Model file for the job. Use its own axes, mm. Face numbers are marked on the shaded views. Coordinates: 2 decimals unless noted, no trailing zeros. Order: outer loops, then holes, each group sorted by start corner. A loop starts at its lowest first (then second) coordinate and runs counter-clockwise, first axis right, second up.
from build123d import *

# Parameters (mm, degrees)
CROQUIS1_W                         = 431.038
CROQUIS1_H                         = 381
BRIDA_BASE1_DEPTH                  = 1.524
CORTAR_EXTRUIR1_REACH              = 289.647
CROQUIS6_W                         = 4.826
CROQUIS6_H                         = 4.826
BRIDA_DE_ARISTA1_STRIP_W           = 9.144
BRIDA_DE_ARISTA1_STRIP_H           = 1.524
BRIDA_DE_ARISTA1_STRIP_CUT_DEPTH   = 426.212
BRIDA_DE_ARISTA1_STRIP_2_W         = 9.144
BRIDA_DE_ARISTA1_STRIP_2_H         = 1.524
BRIDA_DE_ARISTA1_STRIP_CUT_2_DEPTH = 426.212
BRIDA_DE_ARISTA1_STRIP_3_W         = 9.144
BRIDA_DE_ARISTA1_STRIP_3_H         = 1.524
BRIDA_DE_ARISTA1_STRIP_CUT_3_DEPTH = 371.348
BRIDA_DE_ARISTA1_DEPTH             = 426.212
BRIDA_DE_ARISTA1_BEND_DEPTH        = 426.212
BRIDA_DE_ARISTA1_BEND_2_DEPTH      = 371.348
CORTAR_EXTRUIR2_REACH              = 290.088
CROQUIS16_R                        = 3.9624
CROQUIS16_R_2                      = 2.8956
CROQUIS16_R_3                      = 2.413


# Sheet-metal steps are written as plain solids
with BuildPart() as part:
    # Croquis1 → Brida base1 (new body)
    with BuildSketch(Plane.XY):
        Rectangle(CROQUIS1_W, CROQUIS1_H)
    extrude(amount=-BRIDA_BASE1_DEPTH)

    # Croquis6 → Cortar-Extruir1 (cut, up to next)
    with BuildSketch(Plane.XY, mode=Mode.PRIVATE) as cortar_extruir1_sk1:
        with Locations((-213.106, 188.087)):
            Rectangle(CROQUIS6_W, CROQUIS6_H)
    cortar_extruir1_tool1 = extrude(cortar_extruir1_sk1.sketch, amount=-CORTAR_EXTRUIR1_REACH, mode=Mode.PRIVATE) & part.part
    # Croquis6 → Cortar-Extruir1 (cut, up to next)
    with BuildSketch(Plane.XY, mode=Mode.PRIVATE) as cortar_extruir1_sk2:
        with Locations((-213.106, -188.087)):
            Rectangle(CROQUIS6_W, CROQUIS6_H)
    cortar_extruir1_tool2 = extrude(cortar_extruir1_sk2.sketch, amount=-CORTAR_EXTRUIR1_REACH, mode=Mode.PRIVATE) & part.part
    add(cortar_extruir1_tool1.solids().sort_by_distance((-213.106, 188.087, 0))[0], mode=Mode.SUBTRACT)
    add(cortar_extruir1_tool2.solids().sort_by_distance((-213.106, -188.087, 0))[0], mode=Mode.SUBTRACT)

    # Brida de arista1 strip (across the edge) → Brida de arista1 strip cut (cut)
    with BuildSketch(Plane(origin=(-210.693, 190.5, -1.524), x_dir=(0, -1, 0), z_dir=(1, 0, 0))):
        with Locations((-1.524, -0.762)):
            Rectangle(BRIDA_DE_ARISTA1_STRIP_W, BRIDA_DE_ARISTA1_STRIP_H)
    extrude(amount=BRIDA_DE_ARISTA1_STRIP_CUT_DEPTH, mode=Mode.SUBTRACT)

    # Brida de arista1 strip 2 (across the edge) → Brida de arista1 strip cut 2 (cut)
    with BuildSketch(Plane(origin=(215.519, -190.5, -1.524), x_dir=(0, 1, 0), z_dir=(-1, 0, 0))):
        with Locations((-1.524, -0.762)):
            Rectangle(BRIDA_DE_ARISTA1_STRIP_2_W, BRIDA_DE_ARISTA1_STRIP_2_H)
    extrude(amount=BRIDA_DE_ARISTA1_STRIP_CUT_2_DEPTH, mode=Mode.SUBTRACT)

    # Brida de arista1 strip 3 (across the edge) → Brida de arista1 strip cut 3 (cut)
    with BuildSketch(Plane(origin=(-215.519, -185.674, -1.524), x_dir=(1, 0, 0), z_dir=(0, 1, 0))):
        with Locations((-1.524, -0.762)):
            Rectangle(BRIDA_DE_ARISTA1_STRIP_3_W, BRIDA_DE_ARISTA1_STRIP_3_H)
    extrude(amount=BRIDA_DE_ARISTA1_STRIP_CUT_3_DEPTH, mode=Mode.SUBTRACT)

    # Brida de arista1 section (across the edge) → Brida de arista1 (add)
    with BuildSketch(Plane(origin=(-210.693, 190.5, -1.524), x_dir=(0, -1, 0), z_dir=(1, 0, 0))):
        with BuildLine():
            Line((0, 1.524), (0, 14.478))
            Line((0, 14.478), (1.524, 14.478))
            Line((1.524, 14.478), (1.524, 1.524))
            ThreePointArc((1.524, 1.524), (1.970369265, 0.446369265), (3.048, 0))
            Line((3.048, 0), (3.048, -1.524))
            ThreePointArc((3.048, -1.524), (0.892738531, -0.631261469), (0, 1.524))
        make_face()
    extrude(amount=BRIDA_DE_ARISTA1_DEPTH)

    # Brida de arista1 section 2 (across the edge) → Brida de arista1 bend (add)
    with BuildSketch(Plane(origin=(215.519, -190.5, -1.524), x_dir=(0, 1, 0), z_dir=(-1, 0, 0))):
        with BuildLine():
            Line((0, 1.524), (0, 14.478))
            Line((0, 14.478), (1.524, 14.478))
            Line((1.524, 14.478), (1.524, 1.524))
            ThreePointArc((1.524, 1.524), (1.970369265, 0.446369265), (3.048, 0))
            Line((3.048, 0), (3.048, -1.524))
            ThreePointArc((3.048, -1.524), (0.892738531, -0.631261469), (0, 1.524))
        make_face()
    extrude(amount=BRIDA_DE_ARISTA1_BEND_DEPTH)

    # Brida de arista1 section 3 (across the edge) → Brida de arista1 bend 2 (add)
    with BuildSketch(Plane(origin=(-215.519, -185.674, -1.524), x_dir=(1, 0, 0), z_dir=(0, 1, 0))):
        with BuildLine():
            Line((0, 1.524), (0, 14.478))
            Line((0, 14.478), (1.524, 14.478))
            Line((1.524, 14.478), (1.524, 1.524))
            ThreePointArc((1.524, 1.524), (1.970369265, 0.446369265), (3.048, 0))
            Line((3.048, 0), (3.048, -1.524))
            ThreePointArc((3.048, -1.524), (0.892738531, -0.631261469), (0, 1.524))
        make_face()
    extrude(amount=BRIDA_DE_ARISTA1_BEND_2_DEPTH)

    # Croquis16 → Cortar-Extruir2 (cut, up to next)
    with BuildSketch(Plane.XY, mode=Mode.PRIVATE) as cortar_extruir2_sk1:
        with Locations((-202.819, 0)):
            Circle(CROQUIS16_R)
    cortar_extruir2_tool1 = extrude(cortar_extruir2_sk1.sketch, amount=-CORTAR_EXTRUIR2_REACH, mode=Mode.PRIVATE) & part.part
    # Croquis16 → Cortar-Extruir2 (cut, up to next)
    with BuildSketch(Plane.XY, mode=Mode.PRIVATE) as cortar_extruir2_sk2:
        with Locations((-167.767, 60.452)):
            Circle(CROQUIS16_R_2)
    cortar_extruir2_tool2 = extrude(cortar_extruir2_sk2.sketch, amount=-CORTAR_EXTRUIR2_REACH, mode=Mode.PRIVATE) & part.part
    # Croquis16 → Cortar-Extruir2 (cut, up to next)
    with BuildSketch(Plane.XY, mode=Mode.PRIVATE) as cortar_extruir2_sk3:
        with Locations((-167.767, -60.452)):
            Circle(CROQUIS16_R_2)
    cortar_extruir2_tool3 = extrude(cortar_extruir2_sk3.sketch, amount=-CORTAR_EXTRUIR2_REACH, mode=Mode.PRIVATE) & part.part
    # Croquis16 → Cortar-Extruir2 (cut, up to next)
    with BuildSketch(Plane.XY, mode=Mode.PRIVATE) as cortar_extruir2_sk4:
        with Locations((207.645, 152.4)):
            Circle(CROQUIS16_R_3)
    cortar_extruir2_tool4 = extrude(cortar_extruir2_sk4.sketch, amount=-CORTAR_EXTRUIR2_REACH, mode=Mode.PRIVATE) & part.part
    # Croquis16 → Cortar-Extruir2 (cut, up to next)
    with BuildSketch(Plane.XY, mode=Mode.PRIVATE) as cortar_extruir2_sk5:
        with Locations((207.645, 0)):
            Circle(CROQUIS16_R_3)
    cortar_extruir2_tool5 = extrude(cortar_extruir2_sk5.sketch, amount=-CORTAR_EXTRUIR2_REACH, mode=Mode.PRIVATE) & part.part
    # Croquis16 → Cortar-Extruir2 (cut, up to next)
    with BuildSketch(Plane.XY, mode=Mode.PRIVATE) as cortar_extruir2_sk6:
        with Locations((207.645, -152.4)):
            Circle(CROQUIS16_R_3)
    cortar_extruir2_tool6 = extrude(cortar_extruir2_sk6.sketch, amount=-CORTAR_EXTRUIR2_REACH, mode=Mode.PRIVATE) & part.part
    add(cortar_extruir2_tool1.solids().sort_by_distance((-202.819, 0, 0))[0], mode=Mode.SUBTRACT)
    add(cortar_extruir2_tool2.solids().sort_by_distance((-167.767, 60.452, 0))[0], mode=Mode.SUBTRACT)
    add(cortar_extruir2_tool3.solids().sort_by_distance((-167.767, -60.452, 0))[0], mode=Mode.SUBTRACT)
    add(cortar_extruir2_tool4.solids().sort_by_distance((207.645, 152.4, 0))[0], mode=Mode.SUBTRACT)
    add(cortar_extruir2_tool5.solids().sort_by_distance((207.645, 0, 0))[0], mode=Mode.SUBTRACT)
    add(cortar_extruir2_tool6.solids().sort_by_distance((207.645, -152.4, 0))[0], mode=Mode.SUBTRACT)


solid = part.part
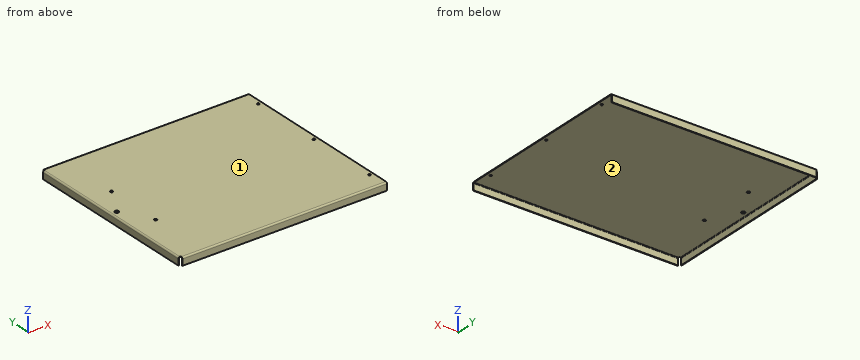
Q1. Mould opens along Y. For the marked faces 1 and 2 say: pulls with the +Y half, pulls with the -Y half, needs draft (parallel to the pull), parting line crosses it, or undercut.
Established:
face 1: needs draft
face 2: undercut
Q2. Probe line 1 (Y direction, x = -140.5, z = -13.75); line 2 (Y direction, x = -53.5, z = -2.5); line 3 (Z direction, x = -113.5, y = 121). List the from-to ranges inside material, lowest first.
Established:
line 1: y = -190.5 to -188.98, 188.98 to 190.5
line 2: y = -190.45 to -188.87, 188.87 to 190.45
line 3: z = -1.52 to 0
Q3. Cut at B-B, the plane y = 21. List the corners of the cut face in (x, z) (3 decimals).
Established:
outline: (-215.519, -16.002) - (-213.995, -16.002) - (-213.995, -3.048) arc R1.524 cw to (-212.471, -1.524) - (215.519, -1.524) - (215.519, 0) - (-212.471, 0) arc R3.048 ccw to (-215.519, -3.048) - close
Q4. Drop flat-ended pins along their axis: P1, Ø6.5, axis at y = 0, z = -10.5, coming from the +X side (3 decimals); P2, Ø7.5, axis at x = 207.645, y = -152.4, coming from the -Z side; P3, Ø5.5, axis at x = -214, z = -4.5, coming from the +Y side. Give the stop position or say it passes through.
Established:
P1: stops at x = -213.995
P2: stops at z = -1.52
P3: stops at y = 185.67
Q5. Cut at C-C, the plane x = 176. List the corners of the cut face in (y, z), plus the area to 3 significant figures.
Established:
outline: (-190.5, -16) - (-188.98, -16) - (-188.98, -3.05) arc R1.52 cw to (-187.45, -1.52) - (187.45, -1.52) arc R1.52 cw to (188.98, -3.05) - (188.98, -16) - (190.5, -16) - (190.5, -3.05) arc R3.05 ccw to (187.45, 0) - (-187.45, 0) arc R3.05 ccw to (-190.5, -3.05) - close
area: 622 mm2
Q6. Cut at A-A, the plane z = -7.75. List the corners of the cut face in (x, y) (3 decimals).
Established:
outline: (-215.519, -185.674) - (-213.995, -185.674) - (-213.995, 185.674) - (-215.519, 185.674) - close; (-210.693, -190.5) - (215.519, -190.5) - (215.519, -188.976) - (-210.693, -188.976) - close; (-210.693, 188.976) - (215.519, 188.976) - (215.519, 190.5) - (-210.693, 190.5) - close
